Autodesk Inventor part; units mm, degrees
ref_plane "YZ Plane" through (0, 0, 0) normal (1, 0, 0) x (0, 1, 0)
ref_plane "XZ Plane" through (0, 0, 0) normal (0, 1, 0) x (-1, 0, 0)
ref_plane "XY Plane" through (0, 0, 0) normal (0, 0, 1) x (1, 0, 0)
sketch "Sketch1" plane through (0, 0, 0) normal (1, 0, 0) x (0, 1, 0)
  line L0 (0, 0) -> (3, 0)
  line L1 (3, 0) -> (3, -23)
  line L2 (3, -23) -> (0, -23)
  line L3 (0, -23) -> (0, 0)
  line L4 (3, -0.8) -> (2.525, -0.8)
  line L5 (2.525, -0.8) -> (2.525, -1.5)
  line L6 (2.525, -1.5) -> (3, -1.5)
  line L7 (3, -1.5) -> (3, -0.8)
  line L8 (3, -22.2) -> (2.525, -22.2)
  line L9 (2.525, -22.2) -> (2.525, -21.5)
  line L10 (2.525, -21.5) -> (3, -21.5)
  line L11 (3, -21.5) -> (3, -22.2)
  point P0 (2.525, -21.85)
  point P1 (3, -21.5)
  point P2 (1.5, -23)
  dimension "d0" = 6
  dimension "d1" = 20
  dimension "d4" = 0.7
  dimension "d5" = 0.7
  dimension "d6" = 5.05
  dimension "d11" = 23
  dimension "d12" = 0.8
revolve "Revolution1" add sketch "Sketch1" angle 360 about axis through (0, 0, -23) along (0, 0, 1) contours L0 L1 L4 L5 L6 L10 L9 L8 L2 L3
chamfer "Chamfer1" distance 0.5 angle 45 2 edges at (0, -3, 0) (0, -3, -23)
equation "\"d5\" = d4"
properties part number "rod pin_CPY"
Model file for the job. Use its own axes, mm. A direction names the side the tool comes from. Round coordinates to 2 decimals unless told otherwise and drop trailing zeros. Order: outer loops, then holes, each group sorted by start corner. A loop starts at its lowest first (then second) coordinate and runs counter-clockwise, first axis right, second up. Notation, with made-up numbers: M -22.5,59 L 34.5,59 A21 cw 34.5,79 Z; hole C 68,-5.5 d3. An arc over 180 degrees is marked long. Use CSV: the item, a comma, the result in double quotes.
Item 1: Pull direction Z, two halves, no side cores. Call faces 1 (the face through (-2.93, -0.65, -0.65)), 2 (the face through (2, -2, -0.8)), 3 (the face through (2, -2, -21.5)), 4 (the face through (0, 0, -23)): released by +Z, released by -Z, zero draft, split by the parting line, or undercut.
Worked answers:
face 1,"zero draft"
face 2,"undercut"
face 3,"undercut"
face 4,"released by -Z"
Item 2: Pin check, flat tips, straight feed: pin 1 (1.5 mm diameter, centred on x = 1.5, z = -15.5, fed in from -Y); pin 2 (1.5 mm diameter, centred on y = 1, z = -15, fed in from -X); pin 3 (2 mm diameter, centred on y = 1.5, z = -4.5, fed in from +X). Stop position of each tip, or through.
Worked answers:
pin 1,"y = -2.9"
pin 2,"x = -2.99"
pin 3,"x = 2.96"
Item 3: Probe probe 1 along Z at (x, y) = (-2.65, -0.25); probe 2 along X at (y, z) = (-0.15, -21.75); probe 3 along Y at (x, z) = (0.15, -8.5). List the from-to ranges inside material, lowest first.
Worked answers:
probe 1,"-22.84 to -22.2, -21.5 to -1.5, -0.8 to -0.16"
probe 2,"-2.52 to 2.52"
probe 3,"-3 to 3"
Item 4: Saw through at A-A (z = -16.25). List the corners of the cut face in (x, y), plus the area to 3 significant figures.
Worked answers:
outline,"C 0,0 d6"
area,"28.3 mm²"
Item 5: Which spindle directions (+Z, -Z, +X, -X, +Y, -Y) get a long thin tool onto all of the face, cutting with end or side? Do faces 5 (the face through (2, -2, -1.5)), 6 (the face through (-2.93, -0.65, -22.35)). Say none if no direction does.
Worked answers:
face 5,"none"
face 6,"+Z, -Z"
